The model under review builds one solid part; all positions refer to its coordinate system, in mm. A direction names the side the tool comes from. Give positions to 0.01 mm unless a question says otherwise; leave off trailing zeros. Order: outer loops, then holes, each group sorted by start corner. A loop starts at its lowest first (then second) coordinate and runs counter-clockwise, first axis right, second up. Notation, with made-up numbers: (62.5, -29.75) -> (92.5, -29.75) arc R11 cw to (92.5, -22.75) -> close; hole circle Ø10 at (62.5, 87). An arc over 180 degrees is marked (long way). Answer as a JSON object with one key per item and string values. Group by question number.
from build123d import *

# Parameters (mm, degrees)
SKETCH1_R           = 3.15
SKETCH1_R_2         = 2.05
BOSS_EXTRUDE1_DEPTH = 13.9
CUT_EXTRUDE1_DEPTH  = 5
CUT_EXTRUDE2_DEPTH  = 4.9
BOSS_EXTRUDE2_DEPTH = 29.1
BOSS_EXTRUDE3_START = 15.2
SKETCH6_R           = 3.15
BOSS_EXTRUDE3_DEPTH = 7.9
BOSS_EXTRUDE4_DEPTH = 6
CUT_EXTRUDE3_DEPTH  = 23
SKETCH9_R           = 2.05
CUT_EXTRUDE4_DEPTH  = 23


with BuildPart() as part:
    # Sketch1 → Boss-Extrude1 (new body)
    with BuildSketch(Plane(origin=(0, 0, 0), x_dir=(0, 0, -1), z_dir=(1, 0, 0))):
        Polygon((0, 0), (14, 0), (14, -5), (-22.167074323, -5), (-26, -2), (-26, 4), (-7.998085585, 27), (-1.998085585, 27), (1.001914415, 24.003735659), (1.001914415, 18.003735659), (-3.00034998, 14), (-3.00034998, 10), (0, 6.5), align=None)
        with Locations((-20, 1.104234986)):
            Circle(SKETCH1_R, mode=Mode.SUBTRACT)
        with Locations((-5, 21)):
            Circle(SKETCH1_R_2, mode=Mode.SUBTRACT)
    extrude(amount=-BOSS_EXTRUDE1_DEPTH)

    # Sketch2 → Cut-Extrude1 (cut)
    with BuildSketch(Plane(origin=(0, 0, 0), x_dir=(0, 0, -1), z_dir=(1, 0, 0))):
        Polygon((-23.651924207, 7), (-13, 7), (-13, -5), (-22.167074323, -5), (-26, -2), (-26, 4), align=None)
    extrude(amount=-CUT_EXTRUDE1_DEPTH, mode=Mode.SUBTRACT)

    # Sketch4 → Cut-Extrude2 (cut)
    with BuildSketch(Plane.ZY.offset(13.9)):
        Polygon((3.00034998, 14), (9.00034998, 14), (10.668359731, 16.093612192), (15.548359731, 17.353453452), (7.998085585, 27), (1.998085585, 27), (-1.001914415, 24.003735659), (-1.001914415, 18.003735659), align=None)
    extrude(amount=-CUT_EXTRUDE2_DEPTH, mode=Mode.SUBTRACT)

    # Sketch5 → Boss-Extrude2 (add)
    with BuildSketch(Plane.ZY.offset(13.9)):
        Polygon((0, 0), (-14, 0), (-14, -5), (5, -5), (5, 6.5), (0, 6.5), align=None)
    extrude(amount=BOSS_EXTRUDE2_DEPTH)

    # Sketch6 → Boss-Extrude3 (add)
    with BuildSketch(Plane.ZY.offset(13.9).offset(BOSS_EXTRUDE3_START)):
        Polygon((5, 6.5), (5, -5), (22.167074323, -5), (26, -2), (26, 4), (23.651924207, 7), align=None)
        with Locations(Location((20, 1.104234986, 0), (0, 0, 180))):
            Circle(SKETCH6_R, mode=Mode.SUBTRACT)
    extrude(amount=BOSS_EXTRUDE3_DEPTH)

    # Sketch7 → Boss-Extrude4 (add)
    with BuildSketch(Plane.ZY.offset(37)):
        Polygon((5, 6.5), (23.651924207, 7), (26, 4), (26, -2), (22.167074323, -5), (5, -5), align=None)
    extrude(amount=BOSS_EXTRUDE4_DEPTH)

    # Sketch8 → Cut-Extrude3 (cut)
    with BuildSketch(Plane(origin=(0, 6.361394216, -0.170529168), x_dir=(1, 0, 0), z_dir=(0, 0.9996408889737135, -0.026797259036029572))):
        Polygon((-37, -26.097852149), (-37, -13.097852149), (-43, -5.097852149), (-43, -26.097852149), align=None)
    extrude(amount=-CUT_EXTRUDE3_DEPTH, mode=Mode.SUBTRACT)

    # Sketch9 → Cut-Extrude4 (cut)
    with BuildSketch(Plane(origin=(0, 0, 0), x_dir=(1, 0, 0), z_dir=(0, 1, 0))):
        with Locations(Location((-21.5, 7, 0), (0, 0, 270))):
            Circle(SKETCH9_R)
        with Locations(Location((-6.5, 7, 0), (0, 0, 270))):
            Circle(SKETCH9_R)
        with Locations(Location((-36.5, 7, 0), (0, 0, 90))):
            Circle(SKETCH9_R)
    extrude(amount=-CUT_EXTRUDE4_DEPTH, mode=Mode.SUBTRACT)


solid = part.part
1. Take a section at D-D on x = -6.5. Give the boundary of the cut face in (y, z), plus the area to 3 significant figures.
2. Take a section at A-A on x = -21.5. Give the boundary of the cut face in (y, z), plus the area to 3 significant figures.
3. Take a section at B-B on z = -7. Give the boundary of the cut face in (x, y).
4. For probe 1 along X at (y, z) = (-1.4, -7); probe 2 along Y at (x, z) = (-2, 5); probe 3 along Z at (x, y) = (-13.5, 1), list the stretches that pass through material, from the lowest coordinate up. Write a range as [from, to].
5. For pin 1 (1.5 mm diameter, centred on x = -16, y = 16, fed in from -Z); pin 2 (5.5 mm diameter, centred on y = 21, z = 5, fed in from -X); pin 3 (12.5 mm diameter, centred on x = -21, y = -1.5, fed in from +Z); pin 4 (2.5 mm diameter, centred on x = -1.5, y = 2, fed in from +Z), all flat-tipped, find the tip position at first contact; note any pin that passes through.
6. Draft analysis for pull direction Y (two halves, no side actions). For faces 1 (the flat face through (-11.48, 15.03, 9.82)), 2 (the flat face through (-21, -5, 0)), 3 (the flat face through (-6.853, 8.274, 1.521)), 4 (the cylindrical face through (-38.533, -2.465, -6.733)), state which applies: pulls with the +Y half, pulls with the -Y half, needs draft (parallel to the pull), parting line crosses it, or undercut.
7. Take a section at C-C on z = 14. Give the boundary of the cut face in (x, y), plus the area to 3 significant figures.
8. Machinability: for faces 5 (the flat face through (-4, 16, 1)), 6 (the flat face through (-5, 1.1, 16.5)), 7 (the flat face through (-4, 21, -1.002)), 8 (the flat face through (-11, 14, 6)), 9 (the flat face through (-21, 1, 5)), which of the approach directions +Z, -Z, +X, -X, +Y, -Y give a long, thin tool a straight path to every point of the face, cutting with its end or side? Answer none if there is none.
Checks:
{
 "1": {"outline": "(-5, -14) -> (0, -14) -> (0, -9.05) -> (-5, -9.05) -> close; (-5, -4.95) -> (0, -4.95) -> (0, 0) -> (6.5, 0) -> (10, 3) -> (14, 3) -> (18, -1) -> (24, -1) -> (27, 2) -> (27, 8) -> (4, 26) -> (-2, 26) -> (-5, 22.17) -> close; hole circle Ø6.3 at (1.1, 20); hole circle Ø4.1 at (21, 5)", "area": "608 mm2"},
 "2": {"outline": "(-5, -14) -> (0, -14) -> (0, -9.05) -> (-5, -9.05) -> close; (-5, -4.95) -> (0, -4.95) -> (0, 0) -> (6.5, 0) -> (6.5, 5) -> (-5, 5) -> close", "area": "107 mm2"},
 "3": {"outline": "(-43, -5) -> (-38.55, -5) -> (-38.55, 0) -> (-43, 0) -> close; (-34.45, -5) -> (-23.55, -5) -> (-23.55, 0) -> (-34.45, 0) -> close; (-19.45, -5) -> (-8.55, -5) -> (-8.55, 0) -> (-19.45, 0) -> close; (-4.45, -5) -> (0, -5) -> (0, 0) -> (-4.45, 0) -> close"},
 "4": {"probe 1": "x = [-43, -38.55], [-34.45, -23.55], [-19.45, -8.55], [-4.45, 0]", "probe 2": "y = [-5, 18.95], [23.05, 27]", "probe 3": "z = [0, 16.85], [23.15, 26]"},
 "5": {"pin 1": "passes through", "pin 2": "stops at x = -9", "pin 3": "stops at z = 5", "pin 4": "stops at z = 13"},
 "6": {"face 1": "pulls with the +Y half", "face 2": "pulls with the -Y half", "face 3": "undercut", "face 4": "needs draft"},
 "7": {"outline": "(-37, -5) -> (-29.1, -5) -> (-29.1, 6.74) -> (-37, 6.74) -> close; (-13.9, -5) -> (-5, -5) -> (-5, 7) -> (0, 7) -> (0, 19.33) -> (-9, 19.33) -> (-9, 16.95) -> (-13.9, 16.95) -> close", "area": "359 mm2"},
 "8": {"face 5": "-Z, +X, -X", "face 6": "+Z, +X, -Y", "face 7": "-Z, +X, -X, +Y", "face 8": "-Z, -X, +Y", "face 9": "+Z, +Y, -Y"}
}
